Source: CAD feature listing. Evaluate the final solid. Frame: model axes, mm. A direction names the side the tool comes from. Round coordinates to 2 decimals unless told otherwise and drop trailing zeros. Order: outer loops, then holes, each group sorted by start corner. A loop starts at its lowest first (then second) coordinate and runs counter-clockwise, first axis right, second up. Notation, with made-up numbers: (2.5, -11) - (10.5, -11) arc R18 cw to (10.5, 1) - close; hole circle Ø9 at (61.25, -25). An arc over 180 degrees is marked (long way). Put each result on its own line as item: value. Start each with the question number.
1) Contact query for a flat-ended pin moving along its axis: P1, Ø1.5, axis at x = 11.5, y = 35.5, coming from the -Z side. Output: stop coordinate, or through.
2) Access query for faces 5 (the face through (37.2, 62.41, 4.44)), 6 (the face through (-1, 1, 10)). Directions: +Z, -Z, +X, -X, +Y, -Y. A direction counts if a zero-diameter tool reaches every point of the face in a straight line with its end or side. Return the directions, or none.
3) Section B-B on y = 11. Output: boundary loops of the cut face in (x, z) (1 decimal).
4) Mould query, pull axis Y, two halves, no side actions, for faces 1 (the face through (-42.075, 1, 4)), 2 (the face through (-37.2, -62.41, 4.44)), 3 (the face through (37.01, -62.6, 4.44)), 4 (the face through (0, 67.475, 4)). Classes: +Y half, -Y half, draft (parallel to the pull), parting line (faces both ways), or undercut.
5) Section C-C on x = -2.5. Output: boundary loops of the cut face in (y, z) (1 decimal).
6) Line query: probe 1 along Y at (x, z) = (8, 5) (3 decimals); probe 2 along X at (y, z) = (-49, 7) (3 decimals); probe 3 along Z at (x, y) = (7, 1.5). Output: solid intervals per line, ascending. Write a range as [from, to].
7) Section A-A on z = 3.5. Output: boundary loops of the cut face in (x, y) (3 decimals), then the cut area to 3 significant figures.
```python
from build123d import *

# Parameters (mm, degrees)
F1_DEPTH = 10
F2_R     = 1.5875
F4_DEPTH = 9


with BuildPart() as f1:
    # F0 (on Top) → F1 (new body)
    with BuildSketch(Plane.XY):
        with BuildLine():
            ThreePointArc((42.0751, 54.7751), (38.355356, 63.755356), (29.3751, 67.4751))
            Line((29.3751, 67.4751), (-29.3751, 67.4751))
            ThreePointArc((-29.3751, 67.4751), (-38.355356, 63.755356), (-42.0751, 54.7751))
            Line((-42.0751, 54.7751), (-42.0751, -54.7751))
            ThreePointArc((-42.0751, -54.7751), (-38.355356, -63.755356), (-29.3751, -67.4751))
            Line((-29.3751, -67.4751), (29.3751, -67.4751))
            ThreePointArc((29.3751, -67.4751), (38.355356, -63.755356), (42.0751, -54.7751))
            Line((42.0751, -54.7751), (42.0751, 54.7751))
        make_face()
    extrude(amount=F1_DEPTH)

    # F2
    f2_edges = [f1.edges().sort_by_distance(p)[0] for p in [
        (42.0751, 0, 10),
        (38.355356, -63.755356, 10),
        (0, -67.4751, 10),
        (-38.355356, -63.755356, 10),
        (-42.0751, 0, 10),
        (-38.355356, 63.755356, 10),
        (0, 67.4751, 10),
        (38.355356, 63.755356, 10),
    ]]
    fillet(f2_edges, radius=F2_R)

    # F3 (on Top) → F4 (cut)
    with BuildSketch(Plane.XY):
        with BuildLine():
            Line((-28.125, -66.225), (28.125, -66.225))
            ThreePointArc((28.125, -66.225), (37.105256, -62.505256), (40.825, -53.525))
            Line((40.825, -53.525), (40.825, 53.525))
            ThreePointArc((40.825, 53.525), (37.105256, 62.505256), (28.125, 66.225))
            Line((28.125, 66.225), (-28.125, 66.225))
            ThreePointArc((-28.125, 66.225), (-37.105256, 62.505256), (-40.825, 53.525))
            Line((-40.825, 53.525), (-40.825, -53.525))
            ThreePointArc((-40.825, -53.525), (-37.105256, -62.505256), (-28.125, -66.225))
        make_face()
    extrude(amount=F4_DEPTH, mode=Mode.SUBTRACT)


solid = f1.part
```
Answer sheet:
1. P1: z = 9
2. face 5: -Z
2. face 6: +Z, +X, -X, +Y, -Y
3. outline: (-42.1, 0) - (-40.8, 0) - (-40.8, 9) - (40.8, 9) - (40.8, 0) - (42.1, 0) - (42.1, 8.4) arc R1.6 ccw to (40.5, 10) - (-40.5, 10) arc R1.6 ccw to (-42.1, 8.4) - close
4. face 1: draft
4. face 2: undercut
4. face 3: undercut
4. face 4: +Y half
5. outline: (-67.5, 0) - (-66.2, 0) - (-66.2, 9) - (66.2, 9) - (66.2, 0) - (67.5, 0) - (67.5, 8.4) arc R1.6 ccw to (65.9, 10) - (-65.9, 10) arc R1.6 ccw to (-67.5, 8.4) - close
6. probe 1: [-67.475, -66.225], [66.225, 67.475]
6. probe 2: [-42.075, -40.825], [40.825, 42.075]
6. probe 3: [9, 10]
7. outline: (-42.075, -54.775) arc R12.7 ccw to (-29.375, -67.475) - (29.375, -67.475) arc R12.7 ccw to (42.075, -54.775) - (42.075, 54.775) arc R12.7 ccw to (29.375, 67.475) - (-29.375, 67.475) arc R12.7 ccw to (-42.075, 54.775) - close; hole (-40.825, -53.525) arc R12.7 ccw to (-28.125, -66.225) - (28.125, -66.225) arc R12.7 ccw to (40.825, -53.525) - (40.825, 53.525) arc R12.7 ccw to (28.125, 66.225) - (-28.125, 66.225) arc R12.7 ccw to (-40.825, 53.525) - close
7. area: 542 mm^2
